Autodesk Inventor part; units mm, degrees
ref_plane "Work Plane1" through (5.9236, 42.877, 6.35) normal (0, -1, 0) x (1, 0, 0)
ref_plane "YZ Plane" through (0, 0, 0) normal (1, 0, 0) x (0, 1, 0)
ref_plane "XZ Plane" through (0, 0, 0) normal (0, 1, 0) x (-1, 0, 0)
sketch "Sketch1" plane through (0, 0, 0) normal (0, 0, 1) x (1, 0, 0)
  line L0 (0, 0) -> (0, 40.5892) construction
  circle A0 centre (0, 40.5892) radius 3.175
  line L1 (0, 0) -> (-19.05, 0)
  arc A1 (5.9236, 42.877) -> (-5.9236, 42.877) centre (0, 40.5892) ccw
  line L2 (-19.05, 0) -> (-19.05, 8.89)
  line L3 (-19.05, 8.89) -> (-5.9236, 42.877)
  line L4 (0, 0) -> (19.05, 0)
  line L5 (19.05, 0) -> (19.05, 8.89)
  line L6 (19.05, 8.89) -> (5.9236, 42.877)
  dimension "d0" = 40.5892
  dimension "d1" = 6.35
  dimension "d3" = 19.05
  dimension "d4" = 12.7
  dimension "d7" = 8.89
extrude "Extrusion1" add sketch "Sketch1" along normal blind 12.7
ref_plane "Work Plane1" through (5.9236, 42.877, 6.35) normal (0, -1, 0) x (1, 0, 0)
sketch "Sketch3" plane through (5.9236, 42.877, 6.35) normal (0, -1, 0) x (1, 0, 0)
  line L0 (3.6014, 6.1842) -> (3.6014, -6.35) construction
  circle A0 centre (3.6014, -0.0829) radius 3.175
  point P0 (-5.9236, -6.35)
  point P1 (3.6014, 6.35)
  point P2 (3.6014, 6.35)
  point P3 (3.6014, 6.35)
  dimension "d12" = 6.35
extrude "Extrusion2" cut sketch "Sketch3" along normal up to surface (33.987 mm away)
mirror "Mirror1" about plane through (0, 0, 0) normal (1, 0, 0) of "Extrusion2"
properties part number "Y_axis_motor_shaft_end_support" material "Aluminum 6061"
Design review of the part built by this model. Coordinates are the model's own, in mm. A direction names the side the tool comes from. Coordinates: 2 decimals unless noted, no trailing zeros. Order: outer loops, then holes, each group sorted by start corner. A loop starts at its lowest first (then second) coordinate and runs counter-clockwise, first axis right, second up. Notation, with made-up numbers: M 50.5,72.5 L 85.5,72.5 A21 ccw 85.5,105.5 Z; hole C 20,24 d4. An arc over 180 degrees is marked long. Answer as a JSON object with one key per item and string values. Group by question number.
1) For pin 1 (7.5 mm diameter, centred on x = 0, y = 40.59, fed in from -Z); pin 2 (4 mm diameter, centred on x = 8.5, z = 6.5, fed in from +Y); pin 3 (4 mm diameter, centred on y = 11.5, z = 10, fed in from +X), all flat-tipped, find the tip position at first contact; note any pin that passes through.
2) Add section D-D, the plane y = 14. Write out the cut boundary in (x, z) (3 decimals), then the cut area to 3 significant figures.
3) Wall thickness on L1, parallel to Y at x = 0, z = 2.75; L2, parallel to X at y = 14, z = 3.5; L3, parallel to X at y = 11.5, z = 5.25: over which ranges is each line inside the solid? List them lowest first.
4) Mouldability with a two-part tool opening along X and no side actions: class faces 3 (the flat face through (14.037, 21.869, 6.261)), 4 (the cylindrical face through (-6.353, 21.953, 6.407)), 5 (the flat face through (-19.05, 4, 6)), 6 (the cylindrical face through (6.353, 21.953, 6.128)) as pulls with the +X half, pulls with the -X half, needs draft (parallel to the pull), parting line crosses it, or undercut.
5) Add section B-B, the plane y = 39. Write out the cut boundary in (x, z) (3 decimals).
6) Tool access review of faces 1 (the cylindrical face through (1.707, 37.912, 6.261)), 2 (the flat face through (9, 8.89, 6)): name each direction out of +Z, -Z, +X, -X, +Y, -Y from which nothing blocks a thin tool from reaching the whole face with its end or side.
7) Add section C-C, the plane z = 4.5. Write out the cut boundary in (x, y) (3 decimals).
8) Add section A-A, the plane x = 0. Write out the cut boundary in (y, z), then the cut area to 3 significant figures.
Computed values:
{
 "1": {"pin 1": "stops at z = 0", "pin 2": "stops at y = 8.89", "pin 3": "stops at x = 18.81"},
 "2": {"outline": "M -17.076,0 L 17.076,0 L 17.076,12.7 L -17.076,12.7 Z; hole C -9.525,6.267 d6.35; hole C 9.525,6.267 d6.35", "area": "370 mm^2"},
 "3": {"L1": "y = 0 to 37.41, 43.76 to 46.94", "L2": "x = -17.08 to -11.08, -7.97 to 7.97, 11.08 to 17.08", "L3": "x = -18.04 to -12.53, -6.52 to 6.52, 12.53 to 18.04"},
 "4": {"face 3": "pulls with the +X half", "face 4": "undercut", "face 5": "pulls with the -X half", "face 6": "undercut"},
 "5": {"outline": "M -7.421,0 L -2.749,0 L -2.749,12.7 L -7.421,12.7 L -7.421,8.645 A3.175 cw -7.421,3.889 Z; M 2.749,0 L 7.421,0 L 7.421,3.889 A3.175 cw 7.421,8.645 L 7.421,12.7 L 2.749,12.7 Z"},
 "6": {"face 1": "+Z, -Z", "face 2": "+Y"},
 "7": {"outline": "M -19.05,0 L 19.05,0 L 19.05,8.89 L 12.163,26.722 L 12.163,8.89 L 6.887,8.89 L 6.887,40.382 L 5.924,42.877 A6.35 ccw -5.924,42.877 L -6.887,40.382 L -6.887,8.89 L -12.163,8.89 L -12.163,26.722 L -19.05,8.89 Z; hole C 0,40.589 d6.35"},
 "8": {"outline": "M 0,0 L 37.41,0 L 37.41,12.7 L 0,12.7 Z; M 43.76,0 L 46.94,0 L 46.94,12.7 L 43.76,12.7 Z", "area": "515 mm^2"}
}
